Drawing for the job (mm, zero at the part's lowest x, y, z). A direction names the side the tool comes from. Give positions to 0.01 mm unless a question says otherwise; leave off trailing zeros. Order: outer loops, then holes, each group sorted by start corner. A loop starts at its lowest first (then second) coordinate and runs counter-clockwise, first axis right, second up. Notation, with made-up numbers: (-37, 30) - (-18, 30) arc R31 cw to (-18, 69) - close; hole circle Ø4 at (20, 69.5). An arc over 180 degrees is marked (long way). Use a Markdown table: item, result.
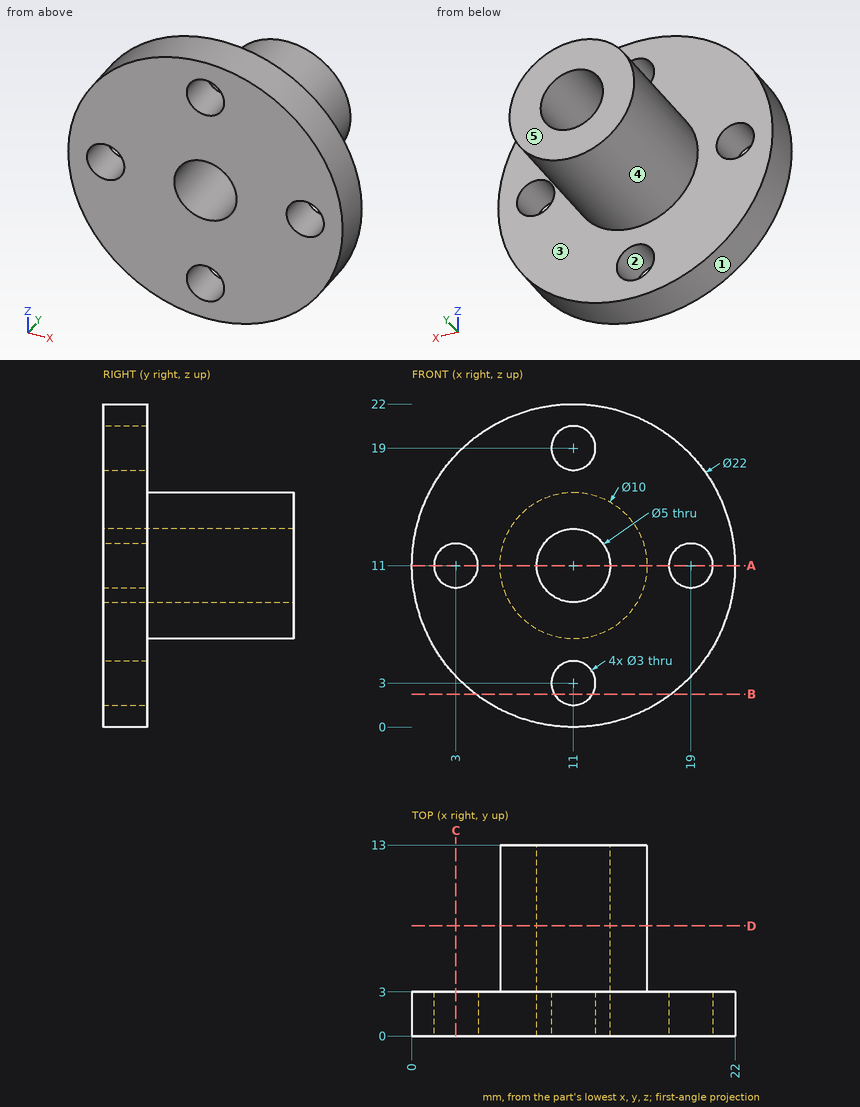
1) Two-plate mould, pull along X, no slides. Class the marked faces 1, 2 and 3: +X half, -X half, draft (parallel to the pull), parting line (faces both ways), or undercut.
Computed:
| item | result |
|---|---|
| face 1 | parting line |
| face 2 | undercut |
| face 3 | draft |
2) Slice it at A-A (z = 11). Write the cut outline in (x, y), and give its area (3 significant figures).
Computed:
| item | result |
|---|---|
| outline | (0, 0) - (1.5, 0) - (1.5, 3) - (0, 3) - close; (4.5, 0) - (8.5, 0) - (8.5, 13) - (6, 13) - (6, 3) - (4.5, 3) - close; (13.5, 0) - (17.5, 0) - (17.5, 3) - (16, 3) - (16, 13) - (13.5, 13) - close; (20.5, 0) - (22, 0) - (22, 3) - (20.5, 3) - close |
| area | 83.0 mm² |
3) Slice it at D-D (y = 7.5). Write the cut outline in (x, z).
Computed:
| item | result |
|---|---|
| outline | circle Ø10 at (11, 11); hole circle Ø5 at (11, 11) |
4) Slice it at C-C (x = 3). Write the cut outline in (y, z), and give its area (3 significant figures).
Computed:
| item | result |
|---|---|
| outline | (0, 3.45) - (3, 3.45) - (3, 9.5) - (0, 9.5) - close; (0, 12.5) - (3, 12.5) - (3, 18.55) - (0, 18.55) - close |
| area | 36.3 mm² |
5) Wall check: line 1 (X direction, y = 1.2, z = 11); line 2 (Y direction, x = 14.5, z = 19); line 3 (X direction, y = 0.95, z = 3). Give the ranges that are in metal, low to high. Write a range as from..to.
Computed:
| item | result |
|---|---|
| line 1 | x = 0..1.5, 4.5..8.5, 13.5..17.5, 20.5..22 |
| line 2 | y = 0..3 |
| line 3 | x = 3.45..9.5, 12.5..18.55 |
6) Tool access for the marked faces 4 and 5: list every direction of +Z, -Z, +X, -X, +Y, -Y with a clear straight run to the whole face (end or side of a thin tool).
Computed:
| item | result |
|---|---|
| face 4 | +Y |
| face 5 | +Z, -Z, +X, -X, +Y |
7) Pin check, flat tips, straight feed: P1, Ø1.5, axis at x = 6.5, y = 6.5, coming from the -Z side; P2, Ø2, axis at x = 15, y = 9.5, coming from the +Z side; P3, Ø1, axis at y = 9.5, z = 13.5, coming from the +X side. Stop position of each tip, or through.
Computed:
| item | result |
|---|---|
| P1 | stops at z = 7.69 |
| P2 | stops at z = 15 |
| P3 | stops at x = 15.58 |
8) Slice it at B-B (z = 2.25). Write the cut outline in (x, y).
Computed:
| item | result |
|---|---|
| outline | (4.33, 0) - (9.7, 0) - (9.7, 3) - (4.33, 3) - close; (12.3, 0) - (17.67, 0) - (17.67, 3) - (12.3, 3) - close |
